Source: three-view drawing plus pictorial views. Frame: mm from the lowest corner of the part. Round coordinates to 2 decimals unless told otherwise and drop trailing zeros. Order: outer loops, then holes, each group sorted by start corner. A loop starts at its lowest first (then second) coordinate and runs counter-clockwise, first axis right, second up. Notation, with made-up numbers: (-11, 5) -> (8, 5) arc R26 cw to (8, 32) -> close; hole circle Ø9 at (70, 35.25). An arc over 180 degrees is marked (long way). Answer as CSV lines item,"result".
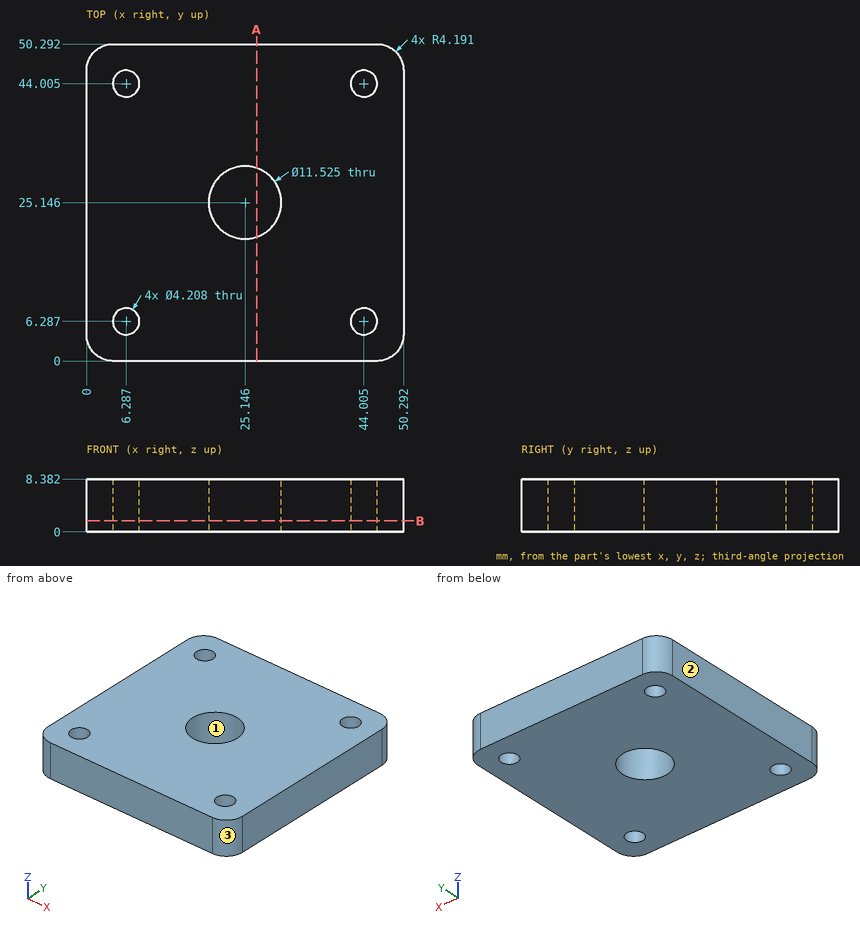
1. Pin query (flat end, axial travel): pin 1 (2.5 mm diameter, centred on x = 44.01, y = 44.01, fed in from +Z). Return the tip coordinate at first contact, or that it passes through.
Results below:
pin 1,"through"
2. Section query A-A on x = 27. Return loops of the section in (y, z).
Results below:
outline,"(0, 0) -> (19.69, 0) -> (19.69, 8.38) -> (0, 8.38) -> close; (30.6, 0) -> (50.29, 0) -> (50.29, 8.38) -> (30.6, 8.38) -> close"
3. Mould query, pull axis Y, two halves, no side actions, for the marked faces 1, 2 and 3. Classes: released by +Y, released by -Y, zero draft, split by the parting line, or undercut.
Results below:
face 1,"undercut"
face 2,"zero draft"
face 3,"released by -Y"
4. Section query B-B on z = 1.75. Return loops of the section in (x, y) (1 decimal).
Results below:
outline,"(0, 4.2) arc R4.2 ccw to (4.2, 0) -> (46.1, 0) arc R4.2 ccw to (50.3, 4.2) -> (50.3, 46.1) arc R4.2 ccw to (46.1, 50.3) -> (4.2, 50.3) arc R4.2 ccw to (0, 46.1) -> close; hole circle Ø4.2 at (6.3, 6.3); hole circle Ø4.2 at (6.3, 44); hole circle Ø11.5 at (25.1, 25.1); hole circle Ø4.2 at (44, 6.3); hole circle Ø4.2 at (44, 44)"
5. Line query: L1, parallel to Y at x = 6.5, z = 0.5; L2, parallel to Y at x = 8, z = 6.5 (1 decimal); L3, parallel to X at y = 28.5, z = 8. Output: solid intervals per line, ascending. Write a range as [from, to].
Results below:
L1,"[0, 4.19], [8.38, 41.91], [46.1, 50.29]"
L2,"[0, 5.1], [7.5, 42.8], [45.2, 50.3]"
L3,"[0, 20.46], [29.83, 50.29]"
